Read the model definition and answer for the solid it produces. Units are mm, in the model's axes. Give positions to 0.01 mm unless a question says otherwise; leave off trailing zeros. Loops run counter-clockwise (first coordinate to the right, second up) from the corner with the lowest first, then second, coordinate; pieces in that order, holes last.
(1) Find section A-A, the plane z = 4. State how many separate pieces and enclosed holes the cut face has, then the cut area to 3 significant figures.
(2) Find section C-C, the plane y = -53.5. Write down the section's boundary in (x, z).
(3) Straight lines are drawn through the part: probe 1 along Y at (x, z) = (0, 8.25); probe 2 along Y at (x, z) = (-151, 3.5); probe 3 along X at (y, z) = (-86, 2). For each, find the intervals that lie inside material, in ascending order.
(4) Find section B-B, the plane x = 36. Write down the section's boundary in (y, z).
(5) Each of these flat-tipped pins is pushed along its axis until it touches: P1, Ø4, axis at x = -18, z = 6, coming from the -Y side; P2, Ø6, axis at y = -108.5, z = 10.5, coming from the -X side; P3, Ø5, axis at y = 85.5, z = 9.5, coming from the -X side; P4, Ø4, axis at x = 0, y = 158.75, coming from the +Z side. Where does it stop, or does it pass through?
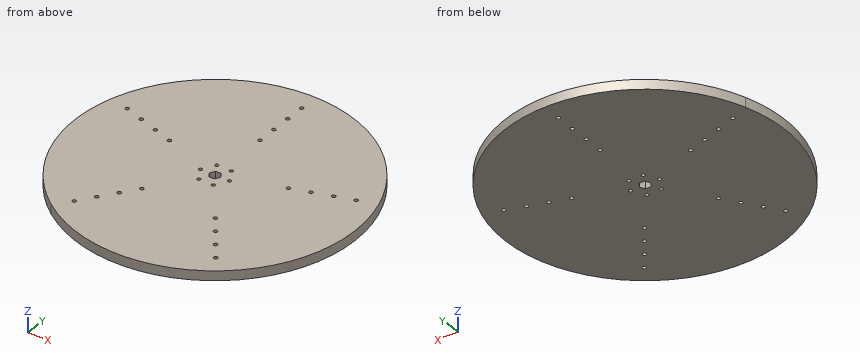
```python
from build123d import *

# Parameters (mm, degrees)
F0_R     = 2.4892
F1_DEPTH = 12.7
F2_R     = 2.286
F3_DEPTH = 12.7


with BuildPart() as f1:
    # F0 (on Top) → F1 (new body)
    with BuildSketch(Plane.XY):
        with BuildLine():
            ThreePointArc((-109.77604, -147.852777), (175.716363, 55.090672), (-174.539009, 58.714197))
            ThreePointArc((-174.539009, 58.714197), (-175.716363, -55.090672), (-109.77604, -147.852777))
        make_face()
        with Locations((-93.310909, -128.431448)):
            Circle(F0_R, mode=Mode.SUBTRACT)
        with Locations((-78.381163, -107.882416)):
            Circle(F0_R, mode=Mode.SUBTRACT)
        with Locations((-63.451418, -87.333385)):
            Circle(F0_R, mode=Mode.SUBTRACT)
        with Locations((-48.521673, -66.784353)):
            Circle(F0_R, mode=Mode.SUBTRACT)
        with Locations((78.381163, -107.882416)):
            Circle(F0_R, mode=Mode.SUBTRACT)
        with Locations((93.310909, -128.431448)):
            Circle(F0_R, mode=Mode.SUBTRACT)
        with Locations((63.451418, -87.333385)):
            Circle(F0_R, mode=Mode.SUBTRACT)
        with Locations((48.521673, -66.784353)):
            Circle(F0_R, mode=Mode.SUBTRACT)
        with Locations((-126.823386, 41.207416)):
            Circle(F0_R, mode=Mode.SUBTRACT)
        with Locations((-102.666551, 33.358385)):
            Circle(F0_R, mode=Mode.SUBTRACT)
        with Locations((-150.980222, 49.056448)):
            Circle(F0_R, mode=Mode.SUBTRACT)
        with Locations((-78.509715, 25.509353)):
            Circle(F0_R, mode=Mode.SUBTRACT)
        with Locations((0, 82.55)):
            Circle(F0_R, mode=Mode.SUBTRACT)
        with Locations((0, 107.95)):
            Circle(F0_R, mode=Mode.SUBTRACT)
        with Locations((0, 133.35)):
            Circle(F0_R, mode=Mode.SUBTRACT)
        with Locations((0, 158.75)):
            Circle(F0_R, mode=Mode.SUBTRACT)
        with Locations((78.509715, 25.509353)):
            Circle(F0_R, mode=Mode.SUBTRACT)
        with Locations((102.666551, 33.358385)):
            Circle(F0_R, mode=Mode.SUBTRACT)
        with Locations((126.823386, 41.207416)):
            Circle(F0_R, mode=Mode.SUBTRACT)
        with Locations((150.980222, 49.056448)):
            Circle(F0_R, mode=Mode.SUBTRACT)
    extrude(amount=F1_DEPTH)

    # F2 (on face) → F3 (cut, through all)
    with BuildSketch(Plane.XY.offset(12.7)):
        Polygon((3.702836, 6.4135), (-3.702836, 6.4135), (-7.405672, 0), (-3.702836, -6.4135), (3.702836, -6.4135), (7.405672, 0), align=None)
        with Locations((-19.05, 0)):
            Circle(F2_R)
        with Locations((-9.525, -16.497784)):
            Circle(F2_R)
        with Locations((9.525, -16.497784)):
            Circle(F2_R)
        with Locations((19.05, 0)):
            Circle(F2_R)
        with Locations((9.525, 16.497784)):
            Circle(F2_R)
        with Locations((-9.525, 16.497784)):
            Circle(F2_R)
    extrude(amount=-F3_DEPTH, mode=Mode.SUBTRACT)


solid = f1.part
```
Entries:
1. separate pieces: 1
1. enclosed holes: 27
1. area: 106,000 mm2
2. outline: (-176.21, 0) - (176.21, 0) - (176.21, 12.7) - (-176.21, 12.7) - close
3. probe 1: y = -184.15 to -6.41, 6.41 to 80.06, 85.04 to 105.46, 110.44 to 130.86, 135.84 to 156.26, 161.24 to 184.15
3. probe 2: y = -105.41 to 46.57, 51.55 to 105.41
3. probe 3: x = -162.83 to -65.55, -61.35 to 61.35, 65.55 to 162.83
4. outline: (-180.6, 0) - (180.6, 0) - (180.6, 12.7) - (-180.6, 12.7) - close
5. P1: stops at y = -183.45
5. P2: stops at x = -150.93
5. P3: stops at x = -164.38
5. P4: passes through
